```python
from build123d import *

# Parameters (mm, degrees)
BOSS_EXTRUDE1_DEPTH = 250
SKETCH2_R           = 19.05
CUT_EXTRUDE1_DEPTH  = 76.2
SKETCH3_R           = 19.05
CUT_EXTRUDE2_DEPTH  = 76.2
SKETCH4_R           = 19.05
CUT_EXTRUDE3_DEPTH  = 76.2


with BuildPart() as part:
    # Sketch1 → Boss-Extrude1 (new body)
    with BuildSketch(Plane.XY):
        Polygon((0, 0), (250, 0), (0, 433.012701892), (-250, 0), align=None)
    extrude(amount=BOSS_EXTRUDE1_DEPTH)

    # Sketch2 → Cut-Extrude1 (cut)
    with BuildSketch(Plane(origin=(187.5, 108.253175473, 0), x_dir=(0, 0, -1), z_dir=(0.866025404, 0.5, 0))):
        with Locations((-125, 125)):
            Circle(SKETCH2_R)
    extrude(amount=-CUT_EXTRUDE1_DEPTH, mode=Mode.SUBTRACT)

    # Sketch3 → Cut-Extrude2 (cut)
    with BuildSketch(Plane.XZ):
        with Locations((0, 125)):
            Circle(SKETCH3_R)
    extrude(amount=-CUT_EXTRUDE2_DEPTH, mode=Mode.SUBTRACT)

    # Sketch4 → Cut-Extrude3 (cut)
    with BuildSketch(Plane(origin=(-187.5, 108.253175473, 0), x_dir=(0, 0, 1), z_dir=(-0.866025404, 0.5, 0))):
        with Locations((125, 125)):
            Circle(SKETCH4_R)
    extrude(amount=-CUT_EXTRUDE3_DEPTH, mode=Mode.SUBTRACT)


solid = part.part
```
Build history of the part. All positions in model axes, mm. A direction names the side the tool comes from. Coordinates: 2 decimals unless noted, no trailing zeros. Write each loop counter-clockwise with the first axis right and the second up, starting at its lowest first coordinate (ties: lowest second). Pieces come first, ordered by that corner, then holes.
1. Drill centre lines: probe 1 along Z at (x, y) = (0, 22.5); probe 2 along Y at (x, z) = (-62.5, 110); probe 3 along Y at (x, z) = (53, 126.5). Where is each one in solid material? Low to high.
Answer block:
probe 1: z = 0 to 105.95, 144.05 to 250
probe 2: y = 0 to 172.36, 193.98 to 324.76
probe 3: y = 0 to 188.81, 196.87 to 341.21
2. Drop flat-ended pins along their axis: pin 1 (6 mm diameter, centred on y = 351.5, z = 93.5, fed in from +X); pin 2 (6 mm diameter, centred on y = 92, z = 93.5, fed in from -X); pin 3 (1 mm diameter, centred on x = 195.5, z = 60, fed in from +Y). Give the stop position or say it passes through.
Answer block:
pin 1: stops at x = 48.79
pin 2: stops at x = -198.62
pin 3: stops at y = 95.26
3. Band-saw the part on A-A, the plane z = 125. Give the cut face in (x, y) (3 decimals), and give its area (3 significant figures).
Answer block:
outline: (-250, 0) - (-19.05, 0) - (-19.05, 76.2) - (19.05, 76.2) - (19.05, 0) - (250, 0) - (134.525, 200.009) - (68.534, 161.909) - (49.484, 194.904) - (115.475, 233.004) - (0, 433.013) - (-115.475, 233.004) - (-49.484, 194.904) - (-68.534, 161.909) - (-134.525, 200.009) - close
area: 99,500 mm2
4. Band-saw the part on C-C, the plane z = 96. Give the cut face in (x, y).
Answer block:
outline: (-250, 0) - (250, 0) - (0, 433.01) - close
5. Band-saw the part on B-B, the plane y = 86. Give the cut face in (x, z), and give its area (3 significant figures).
Answer block:
outline: (-200.35, 0) - (200.35, 0) - (200.35, 250) - (-200.35, 250) - close
area: 100,000 mm2
6. 3-axis set-ups, long thin cutter, end or side, ignore diameter. For faces 1 (the flat face through (58.876, 178.637, 125.267)), 2 (the flat face through (0, 76.2, 125)), 3 (the flat face through (-4, 171, 0)): which of +Z, -Z, +X, -X, +Y, -Y reach the whole face in a straight line?
Answer block:
face 1: none
face 2: -Y
face 3: -Z, +X, -X, +Y, -Y
7. Pull direction X, two halves, no side cores. Call faces 4 (the flat face through (-4, 171, 250)), 5 (the flat face through (126.75, 213.475, 95.472)), 6 (the cylindrical face through (-89.61, 202.68, 143.17)): released by +X, released by -X, zero draft, split by the parting line, or undercut.
Answer block:
face 4: zero draft
face 5: released by +X
face 6: undercut
